Here's how the part is built. I have some questions about the finished solid (model axes, mm). A direction names the side the tool comes from. Round coordinates to 2 decimals unless told otherwise and drop trailing zeros. Write each loop counter-clockwise with the first axis right and the second up, starting at its lowest first coordinate (ties: lowest second). Pieces come first, ordered by that corner, then holes. Notation, with made-up numbers: (62, 47) - (109, 47) arc R28 cw to (109, 70) - close; hole circle Ø10 at (2, 16.5). An arc over 180 degrees is marked (long way). One line per item, written item: value. Start each with the question number.
Item 1: Imagine slicing it at D-D, the plane z = 77. Please give me the cut outline in (x, y), then the cut area to 3 significant figures.
Item 2: Imagine slicing it at A-A, the plane x = 300. Please give me the cut outline in (y, z), then the cut area to 3 significant figures.
Item 3: If I drill on line 1 (X direction, y = 143.5, z = -28); line 2 (Y direction, x = 284, z = -73.5); line 3 (X direction, y = -134.5, z = 18), over which ranges is the centre line in solid material (lowest first)?
Item 4: Imagine slicing it at C-C, the plane z = 0. Please give me the cut outline in (x, y).
Item 5: For faces 1 (the face through (235, -108, 65)), 2 (the face through (310, 145, 1)), 3 (the face through (365, -106, -65)), 4 (the face through (100, 19, 19)), which set-ups out of +Z, -Z, +X, -X, +Y, -Y let a thin tool reach every point of the face, with its end or its side?
Item 6: For P1, Ø3, axis at y = 131, z = -41, coming from the +X side; P2, Ø10, axis at x = 437.5, z = 55, coming from the -Y side; P3, Ø10, axis at x = 303, z = -10, coming from the +Y side, each with a flat end and sliding along its axis, tell me the tip position at first contact or that it passes through.
Item 7: Imagine slicing it at B-B, the plane y = -166. Please give me the cut outline in (x, z).
Item 8: Thinking about a two-plate mould opening in X: for faces 5 (the face through (250.425, -219.37, -6.509)), 6 (the face through (300, 115, -1)), 7 (the face through (365, -106, 65)), 8 (the face through (235, 106, 65)), which applies, released by +X, released by -X, zero draft, split by the parting line, or undercut?
```python
from build123d import *

# Parameters (mm, degrees)
SKETCH4_W           = 180
SKETCH4_H           = 180
BOSS_EXTRUDE2_DEPTH = 175
SKETCH5_R           = 50
BOSS_EXTRUDE3_DEPTH = 90
CHAMFER1_SIZE       = 50
SKETCH6_W           = 20
SKETCH6_H           = 180
CUT_EXTRUDE1_DEPTH  = 60


with BuildPart() as part:
    # Sketch3 → Revolve1 (revolve)
    with BuildSketch(Plane.XY, mode=Mode.PRIVATE) as revolve1_sk:
        Polygon((0, 0), (0, 25), (100, 25), (100, 90), (500, 90), (500, 25), (600, 25), (600, 0), align=None)
    revolve(revolve1_sk.sketch.rotate(Axis((0, 0, 0), (-1, 0, 0)), 90), axis=Axis((0, 0, 0), (-1, 0, 0)))

    # Sketch4 → Boss-Extrude2 (add, symmetric)
    with BuildSketch(Plane(origin=(0, 0, 0), x_dir=(1, 0, 0), z_dir=(0, 1, 0))):
        with Locations((300, 0)):
            Rectangle(SKETCH4_W, SKETCH4_H)
    extrude(amount=BOSS_EXTRUDE2_DEPTH, both=True)

    # Sketch5 → Boss-Extrude3 (add)
    with BuildSketch(Plane.XZ.offset(175)):
        with Locations(Location((300, 0, 0), (0, 0, 90))):
            Circle(SKETCH5_R)
    extrude(amount=BOSS_EXTRUDE3_DEPTH)

    # Chamfer1
    # the kernel refuses this chamfer: 50 mm, written as the material it takes off along each edge
    with BuildSketch(Plane(origin=(210, -303.584149398, -90), x_dir=(-0.027495876610586594, 0, 0.9996219169112966), z_dir=(0, 1, 0))) as chamfer1_piece_1_section:
        Polygon((CHAMFER1_SIZE * 0.999621916911, CHAMFER1_SIZE * 0.0274958766106), (-CHAMFER1_SIZE * 0.0274958766106, CHAMFER1_SIZE * 0.999621916911), (0, 0), align=None)
    chamfer1_piece_1 = extrude(amount=303.584149398, mode=Mode.PRIVATE)
    chamfer1_piece_1 = chamfer1_piece_1 - Plane(origin=(227.472268945, 0, 0), x_dir=(0, 0, -1), z_dir=(1, 0, 0)) * Cylinder(90, 808, mode=Mode.PRIVATE)
    add(chamfer1_piece_1, mode=Mode.SUBTRACT)
    with BuildSketch(Plane(origin=(210, -303.584149398, 90), x_dir=(-0.027495876610586598, 0, -0.9996219169112966), z_dir=(0, 1, 0))) as chamfer1_piece_2_section:
        Polygon((CHAMFER1_SIZE * 0.999621916911, -CHAMFER1_SIZE * 0.0274958766106), (-CHAMFER1_SIZE * 0.0274958766106, -CHAMFER1_SIZE * 0.999621916911), (0, 0), align=None)
    chamfer1_piece_2 = extrude(amount=303.584149398, mode=Mode.PRIVATE)
    chamfer1_piece_2 = chamfer1_piece_2 - Plane(origin=(227.472268938, 0, 0), x_dir=(0, 0, -1), z_dir=(1, 0, 0)) * Cylinder(90, 808, mode=Mode.PRIVATE)
    add(chamfer1_piece_2, mode=Mode.SUBTRACT)
    with BuildSketch(Plane(origin=(390, 0, 90), x_dir=(-0.9996219169112966, 0, 0.02749587661058631), z_dir=(0, -1, 0))) as chamfer1_piece_3_section:
        Polygon((CHAMFER1_SIZE * 0.999621916911, CHAMFER1_SIZE * 0.0274958766106), (-CHAMFER1_SIZE * 0.0274958766106, CHAMFER1_SIZE * 0.999621916911), (0, 0), align=None)
    chamfer1_piece_3 = extrude(amount=303.584149398, mode=Mode.PRIVATE)
    chamfer1_piece_3 = chamfer1_piece_3 - Plane(origin=(372.527731062, 0, 0), x_dir=(0, 0, -1), z_dir=(1, 0, 0)) * Cylinder(90, 808, mode=Mode.PRIVATE)
    add(chamfer1_piece_3, mode=Mode.SUBTRACT)
    with BuildSketch(Plane(origin=(390, 303.584149398, -90), x_dir=(-0.9996219169112966, 0, -0.02749587661058631), z_dir=(0, -1, 0))) as chamfer1_piece_4_section:
        Polygon((CHAMFER1_SIZE * 0.999621916911, -CHAMFER1_SIZE * 0.0274958766106), (-CHAMFER1_SIZE * 0.0274958766106, -CHAMFER1_SIZE * 0.999621916911), (0, 0), align=None)
    chamfer1_piece_4 = extrude(amount=303.584149398, mode=Mode.PRIVATE)
    chamfer1_piece_4 = chamfer1_piece_4 - Plane(origin=(372.527731055, 0, 0), x_dir=(0, 0, -1), z_dir=(1, 0, 0)) * Cylinder(90, 808, mode=Mode.PRIVATE)
    add(chamfer1_piece_4, mode=Mode.SUBTRACT)
    with BuildSketch(Plane(origin=(210, 0, -90), x_dir=(-0.027495876610586594, 0, 0.9996219169112966), z_dir=(0, 1, 0))) as chamfer1_piece_5_section:
        Polygon((CHAMFER1_SIZE * 0.999621916911, CHAMFER1_SIZE * 0.0274958766106), (-CHAMFER1_SIZE * 0.0274958766106, CHAMFER1_SIZE * 0.999621916911), (0, 0), align=None)
    chamfer1_piece_5 = extrude(amount=303.584149398, mode=Mode.PRIVATE)
    chamfer1_piece_5 = chamfer1_piece_5 - Plane(origin=(227.472268945, 0, 0), x_dir=(0, 0, -1), z_dir=(1, 0, 0)) * Cylinder(90, 808, mode=Mode.PRIVATE)
    add(chamfer1_piece_5, mode=Mode.SUBTRACT)
    with BuildSketch(Plane(origin=(210, 0, 90), x_dir=(-0.027495876610586598, 0, -0.9996219169112966), z_dir=(0, 1, 0))) as chamfer1_piece_6_section:
        Polygon((CHAMFER1_SIZE * 0.999621916911, -CHAMFER1_SIZE * 0.0274958766106), (-CHAMFER1_SIZE * 0.0274958766106, -CHAMFER1_SIZE * 0.999621916911), (0, 0), align=None)
    chamfer1_piece_6 = extrude(amount=303.584149398, mode=Mode.PRIVATE)
    chamfer1_piece_6 = chamfer1_piece_6 - Plane(origin=(227.472268947, 0, 0), x_dir=(0, 0, -1), z_dir=(1, 0, 0)) * Cylinder(90, 808, mode=Mode.PRIVATE)
    add(chamfer1_piece_6, mode=Mode.SUBTRACT)
    with BuildSketch(Plane(origin=(390, 303.584149398, 90), x_dir=(-0.9996219169112966, 0, 0.02749587661058631), z_dir=(0, -1, 0))) as chamfer1_piece_7_section:
        Polygon((CHAMFER1_SIZE * 0.999621916911, CHAMFER1_SIZE * 0.0274958766106), (-CHAMFER1_SIZE * 0.0274958766106, CHAMFER1_SIZE * 0.999621916911), (0, 0), align=None)
    chamfer1_piece_7 = extrude(amount=303.584149398, mode=Mode.PRIVATE)
    chamfer1_piece_7 = chamfer1_piece_7 - Plane(origin=(372.527731053, 0, 0), x_dir=(0, 0, -1), z_dir=(1, 0, 0)) * Cylinder(90, 808, mode=Mode.PRIVATE)
    add(chamfer1_piece_7, mode=Mode.SUBTRACT)
    with BuildSketch(Plane(origin=(390, 0, -90), x_dir=(-0.9996219169112966, 0, -0.02749587661058631), z_dir=(0, -1, 0))) as chamfer1_piece_8_section:
        Polygon((CHAMFER1_SIZE * 0.999621916911, -CHAMFER1_SIZE * 0.0274958766106), (-CHAMFER1_SIZE * 0.0274958766106, -CHAMFER1_SIZE * 0.999621916911), (0, 0), align=None)
    chamfer1_piece_8 = extrude(amount=303.584149398, mode=Mode.PRIVATE)
    chamfer1_piece_8 = chamfer1_piece_8 - Plane(origin=(372.527731055, 0, 0), x_dir=(0, 0, -1), z_dir=(1, 0, 0)) * Cylinder(90, 808, mode=Mode.PRIVATE)
    add(chamfer1_piece_8, mode=Mode.SUBTRACT)

    # Sketch6 → Cut-Extrude1 (cut)
    with BuildSketch(Plane(origin=(0, 175, 0), x_dir=(1, 0, 0), z_dir=(0, 1, 0))):
        with Locations((300, 0)):
            Rectangle(SKETCH6_W, SKETCH6_H)
    extrude(amount=-CUT_EXTRUDE1_DEPTH, mode=Mode.SUBTRACT)


solid = part.part
```
Values follow:
1. outline: (100, -46.59) - (247, -46.59) - (247, -175) - (353, -175) - (353, -46.59) - (500, -46.59) - (500, 46.59) - (353, 46.59) - (353, 175) - (310, 175) - (310, 115) - (290, 115) - (290, 175) - (247, 175) - (247, 46.59) - (100, 46.59) - close
1. area: 63,300 mm^2
2. outline: (-265, -50) - (-175, -50) - (-175, -90) - (115, -90) - (115, 90) - (-175, 90) - (-175, 50) - (-265, 50) - close
2. area: 61,200 mm^2
3. line 1: x = 210 to 290, 310 to 390
3. line 2: y = -175 to 175
3. line 3: x = 210 to 390
4. outline: (0, -25) - (100, -25) - (100, -90) - (210, -90) - (210, -175) - (250, -175) - (250, -265) - (350, -265) - (350, -175) - (390, -175) - (390, -90) - (500, -90) - (500, -25) - (600, -25) - (600, 25) - (500, 25) - (500, 90) - (390, 90) - (390, 175) - (310, 175) - (310, 115) - (290, 115) - (290, 175) - (210, 175) - (210, 90) - (100, 90) - (100, 25) - (0, 25) - close
5. face 1: +Z, -X, -Y
5. face 2: +Z, -Z, +Y
5. face 3: -Z, +X, -Y
5. face 4: -X
6. P1: stops at x = 390
6. P2: stops at y = -74.83
6. P3: stops at y = 115
7. outline: (210, -40) - (260, -90) - (340, -90) - (390, -40) - (390, 40) - (340, 90) - (260, 90) - (210, 40) - close
8. face 5: split by the parting line
8. face 6: undercut
8. face 7: released by +X
8. face 8: released by -X
